```python
from build123d import *

# Parameters (mm, degrees)
F0_R     = 1.5
F0_R_2   = 9.525
F1_DEPTH = 6.35
F2_SIZE  = 1.5875
F3_R     = 12.7
F3_R_2   = 9.525
F4_DEPTH = 6.35
F5_SIZE  = 1.5875


with BuildPart() as f1:
    # F0 (on Top) → F1 (new body)
    with BuildSketch(Plane.XY):
        with BuildLine():
            Line((-17.974874, 13.025126), (-11.10737, 6.157623))
            ThreePointArc((-11.10737, 6.157623), (-12.7, 0), (-11.10737, -6.157623))
            Line((-11.10737, -6.157623), (-17.974874, -13.025126))
            ThreePointArc((-17.974874, -13.025126), (-17.974874, -17.974874), (-13.025126, -17.974874))
            Line((-13.025126, -17.974874), (-6.157623, -11.10737))
            ThreePointArc((-6.157623, -11.10737), (0, -12.7), (6.157623, -11.10737))
            Line((6.157623, -11.10737), (13.025126, -17.974874))
            ThreePointArc((13.025126, -17.974874), (17.974874, -17.974874), (17.974874, -13.025126))
            Line((17.974874, -13.025126), (11.10737, -6.157623))
            ThreePointArc((11.10737, -6.157623), (12.7, 0), (11.10737, 6.157623))
            Line((11.10737, 6.157623), (17.974874, 13.025126))
            ThreePointArc((17.974874, 13.025126), (17.974874, 17.974874), (13.025126, 17.974874))
            Line((13.025126, 17.974874), (6.157623, 11.10737))
            ThreePointArc((6.157623, 11.10737), (0, 12.7), (-6.157623, 11.10737))
            Line((-6.157623, 11.10737), (-13.025126, 17.974874))
            ThreePointArc((-13.025126, 17.974874), (-17.974874, 17.974874), (-17.974874, 13.025126))
        make_face()
        with Locations((-15.5, -15.5)):
            Circle(F0_R, mode=Mode.SUBTRACT)
        with Locations((15.5, -15.5)):
            Circle(F0_R, mode=Mode.SUBTRACT)
        with Locations((-15.5, 15.5)):
            Circle(F0_R, mode=Mode.SUBTRACT)
        Circle(F0_R_2, mode=Mode.SUBTRACT)
        with Locations((15.5, 15.5)):
            Circle(F0_R, mode=Mode.SUBTRACT)
    extrude(amount=F1_DEPTH)

    # F2
    f2_edges = [f1.edges().sort_by_distance(p)[0] for p in [
        (-17, -15.5, 0),
        (14, -15.5, 0),
        (14, 15.5, 0),
        (-17, 15.5, 0),
    ]]
    chamfer(f2_edges, length=F2_SIZE)

    # F3 (on face) → F4 (join)
    with BuildSketch(Plane.XY.offset(6.35)):
        Circle(F3_R)
        Circle(F3_R_2, mode=Mode.SUBTRACT)
    extrude(amount=F4_DEPTH)

    # F5
    f5_edges = [f1.edges().sort_by_distance(p)[0] for p in [
        (-12.7, 0, 12.7),
    ]]
    chamfer(f5_edges, length=F5_SIZE)


solid = f1.part
```
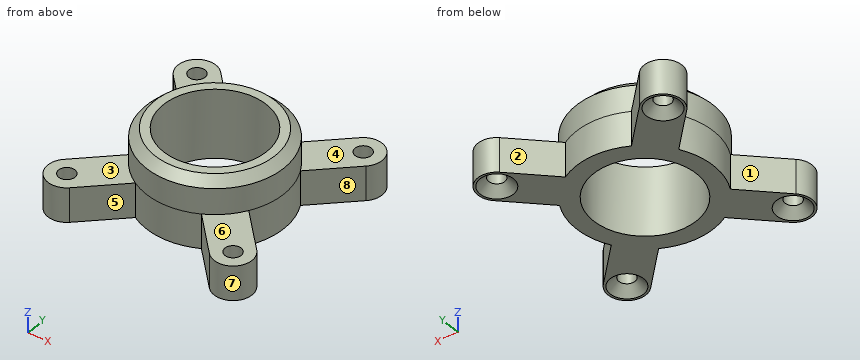
Input: part model. Units: mm. Frame: model coordinates. Face numbers are marked on the shaded views. A direction names the side the tool comes from. Coordinates: 2 decimals unless noted, no trailing zeros. Write each loop counter-clockwise with the first axis right and the second up, starting at its lowest first coordinate (ties: lowest second). Pieces come first, ordered by that corner, then holes.
1) Set-up query: the marked faces 4, 5, 6, 7 and 8. Return all of +Z, -Z, +X, -X, +Y, -Y with unobstructed straight access to the full face (end or side cutting, diameter ignored); none if empty.
2) Material intervals for line 1 along Y through (x, z) = (15.5, 4.45); line 2 along Y through (x, z) = (-16, 2.75); line 3 along X through (y, z) = (-2, 0.5), sorted ascending.
3) Pin query (flat end, axial travel): pin 1 Ø3 at (x, z) = (4.5, 4.5) entering from +Y; pin 2 Ø3.5 at (x, y) = (15.5, -15.5) entering from -Z; pin 3 Ø4 at (x, y) = (-11.5, 15.5) entering from +Z. Return the tip coordinate at first contact, or that it passes through.
4) Mould query, pull axis X, two halves, no side actions, for the marked faces 1, 2 and 3. Classes: pulls with the +X half, pulls with the -X half, needs draft (parallel to the pull), parting line crosses it, or undercut.
5) Section A-A on z = 2.25. Output: boundary loops of the cut face in (x, y) (3 decimals).
6) Section B-B on y = 0. Output: boundary loops of the cut face in (x, z) (1 decimal).
7) Section C-C on x = 15.5. Output: boundary loops of the cut face in (y, z), and give its area (3 significant figures).
Check result:
1. face 4: +Z, +X, +Y
1. face 5: +Z, -Z, -Y
1. face 6: +Z, +X, -Y
1. face 7: +Z, -Z
1. face 8: +Z, -Z, +X
2. line 1: y = -19 to -17, -14 to -10.55, 10.55 to 14, 17 to 19
2. line 2: y = -18.96 to -16.91, -14.09 to -11.05, 11.05 to 14.09, 16.91 to 18.96
2. line 3: x = -12.54 to -9.31, 9.31 to 12.54
3. pin 1: stops at y = 12.34
3. pin 2: stops at z = 1.34
3. pin 3: stops at z = 6.35
4. face 1: pulls with the -X half
4. face 2: undercut
4. face 3: needs draft
5. outline: (-17.975, -13.025) arc R3.5 ccw to (-13.025, -17.975) - (-6.158, -11.107) arc R12.7 ccw to (6.158, -11.107) - (13.025, -17.975) arc R3.5 ccw to (17.975, -13.025) - (11.107, -6.158) arc R12.7 ccw to (11.107, 6.158) - (17.975, 13.025) arc R3.5 ccw to (13.025, 17.975) - (6.158, 11.107) arc R12.7 ccw to (-6.158, 11.107) - (-13.025, 17.975) arc R3.5 ccw to (-17.975, 13.025) - (-11.107, 6.158) arc R12.7 ccw to (-11.107, -6.158) - close; hole circle Ø3 at (-15.5, -15.5); hole circle Ø3 at (-15.5, 15.5); hole circle Ø19.05 at (0, 0); hole circle Ø3 at (15.5, -15.5); hole circle Ø3 at (15.5, 15.5)
6. outline: (-12.7, 0) - (-9.5, 0) - (-9.5, 12.7) - (-11.1, 12.7) - (-12.7, 11.1) - close; (9.5, 0) - (12.7, 0) - (12.7, 11.1) - (11.1, 12.7) - (9.5, 12.7) - close
7. outline: (-19, 0) - (-18.59, 0) - (-17, 1.59) - (-17, 6.35) - (-19, 6.35) - close; (-14, 1.59) - (-12.41, 0) - (-10.55, 0) - (-10.55, 6.35) - (-14, 6.35) - close; (10.55, 0) - (12.41, 0) - (14, 1.59) - (14, 6.35) - (10.55, 6.35) - close; (17, 1.59) - (18.59, 0) - (19, 0) - (19, 6.35) - (17, 6.35) - close
7. area: 64.2 mm2
